Could you check a few things on this model? Use its own coordinates, in mm. Face numbers are marked on the shaded views. A direction names the side the tool comes from. Give positions to 0.01 mm unless a question says otherwise; leave off trailing zeros. Write each loop counter-clockwise with the first axis right and the second up, starting at its lowest first coordinate (ties: lowest second). Pieces come first, ordered by that corner, then holes. Notation, with made-up numbers: (86, 87.25) -> (131, 87.25) arc R25 cw to (131, 117.25) -> close; hole circle Ø8 at (32.5, 25.25). An arc over 180 degrees is marked (long way). Write item = value, one per line. Start each with the question number.
```python
from build123d import *

# Parameters (mm, degrees)
F1_DEPTH = 50.8
F2_R     = 12.7
F3_R     = 12.7
F4_R     = 12.7
F7_D     = 12.7


with BuildPart() as f1:
    # F0 (on Top) → F1 (new body)
    with BuildSketch(Plane.XY):
        Polygon((0, 50.8), (0, 0), (152.4, 0), (152.4, 76.2), (101.6, 76.2), (101.6, 50.8), align=None)
    extrude(amount=F1_DEPTH)

    # F2
    f2_edges = [f1.edges().sort_by_distance(p)[0] for p in [
        (152.4, 76.2, 25.4),
    ]]
    fillet(f2_edges, radius=F2_R)

    # F3
    f3_edges = [f1.edges().sort_by_distance(p)[0] for p in [
        (0, 50.8, 25.4),
    ]]
    fillet(f3_edges, radius=F3_R)

    # F4
    f4_edges = [f1.edges().sort_by_distance(p)[0] for p in [
        (0, 0, 25.4),
        (152.4, 0, 25.4),
    ]]
    fillet(f4_edges, radius=F4_R)

    # F7 (through all)
    with Locations(Plane.XY.offset(50.8)):
        with Locations((29.908501, 25.3365), (81.15299, 25.3365)):
            Hole(F7_D / 2)


solid = f1.part
```
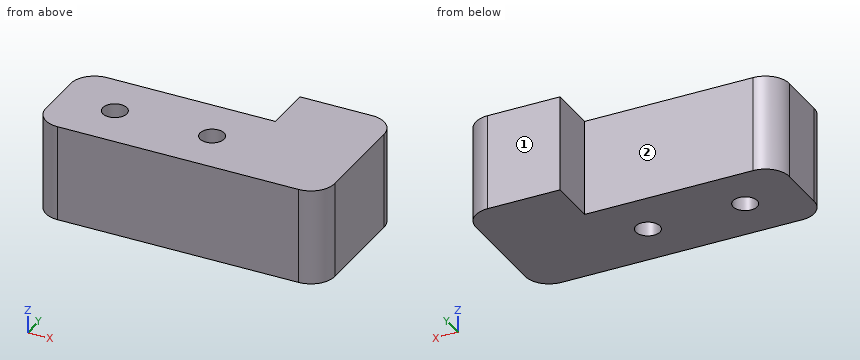
(1) Imagine slicing it at C-C (x = 30.5). Please give me the cut outline in (y, z).
(2) Imagine slicing it at B-B (y = 21). Please give me the cut outline in (x, z).
(3) If I drill on line 1 along X through (y, z) = (25.5, 32); line 2 along X through (y, z) = (30.5, 44.5); line 3 along Y through (x, z) = (93.5, 2), over which ranges is the centre line in solid material (lowest first)? Write a range as from..to.
(4) On a 3-axis mill with a long thin cutter (end or side, diameter ignored), from which of +Z, -Z, +X, -X, +Y, -Y can I reach the whole of each face in a straight line? I mean the marked faces 1 and 2. Say none if no direction works.
(5) I'm going to push flat-ended pins straight in: pin 1 (20.5 mm diameter, centred on y = 63.5, z = 20, fed in from -X); pin 2 (10 mm diameter, centred on x = 19, z = 31, fed in from +Y); pin 3 (12 mm diameter, centred on y = 52.5, z = 6, fed in from -X); pin 4 (7.5 mm diameter, centred on x = 81.15, y = 25.34, fed in from -Z). Where does each tip first touch, or does it pass through?
(6) Imagine slicing it at D-D (y = 48). Please give me the cut outline in (x, z).
(7) Imagine slicing it at A-A (z = 27). Please give me the cut outline in (x, y).
Answers below:
q1.outline = (0, 0) -> (19.01, 0) -> (19.01, 50.8) -> (0, 50.8) -> close; (31.66, 0) -> (50.8, 0) -> (50.8, 50.8) -> (31.66, 50.8) -> close
q2.outline = (0, 0) -> (25.27, 0) -> (25.27, 50.8) -> (0, 50.8) -> close; (34.55, 0) -> (76.51, 0) -> (76.51, 50.8) -> (34.55, 50.8) -> close; (85.79, 0) -> (152.4, 0) -> (152.4, 50.8) -> (85.79, 50.8) -> close
q3.line_1 = 0..23.56, 36.26..74.81, 87.5..152.4
q3.line_2 = 0..26.21, 33.6..77.46, 84.85..152.4
q3.line_3 = 0..50.8
q4.face_1 = +Z, -Z, +X, -X, +Y
q4.face_2 = +Z, -Z, -X, +Y
q5.pin_1 = 101.6
q5.pin_2 = 50.8
q5.pin_3 = 3.17
q5.pin_4 = through
q6.outline = (4.75, 0) -> (152.4, 0) -> (152.4, 50.8) -> (4.75, 50.8) -> close
q7.outline = (0, 12.7) arc R12.7 ccw to (12.7, 0) -> (139.7, 0) arc R12.7 ccw to (152.4, 12.7) -> (152.4, 63.5) arc R12.7 ccw to (139.7, 76.2) -> (101.6, 76.2) -> (101.6, 50.8) -> (12.7, 50.8) arc R12.7 ccw to (0, 38.1) -> close; hole circle Ø12.7 at (29.91, 25.34); hole circle Ø12.7 at (81.15, 25.34)
